The model under review builds one solid part; all positions refer to its coordinate system, in mm. Face numbers are marked on the shaded views. A direction names the side the tool comes from. Round coordinates to 2 decimals unless told otherwise and drop trailing zeros. Loops run counter-clockwise (first coordinate to the right, second up) from the corner with the lowest first, then second, coordinate; pieces in that order, holes last. Notation, with made-up numbers: M 30,84 L 36,84 A12 ccw 36,97 Z; hole C 69.5,51 d7. An arc over 180 degrees is marked long. Answer as a JSON object with one key per item and string values. Group by question number.
Item 1: Consider section A-A (y = 602.5). Give the boundary of the cut face in (x, z) (3 decimals), and give its area (3 significant figures).
Item 2: Consider section B-B (x = 34). Give the boundary of the cut face in (y, z), and give its area (3 significant figures).
Item 3: Insertion check: P1, Ø12, axis at y = -65, z = 20.5, coming from the +X side; P2, Ø1, axis at x = 56, y = 203, coming from the +Z side. Each pin has a flat end and moves straight along its axis. Give the tip position at first contact, or say it passes through.
Item 4: Tool access review of the marked faces 1 and 2: name each direction out of +Z, -Z, +X, -X, +Y, -Y from which nothing blocks a thin tool from reaching the whole face with its end or side.
Item 5: To check wall thickness, follow line 1 (Z direction, x = 1, y = -304); line 2 (X direction, y = 101.6, z = 4); line 3 (X direction, y = -406.4, z = 4.25). State the ranges of each line that lie inside material, in increasing order.
```python
from build123d import *

# Parameters (mm, degrees)
F1_DEPTH = 1066.8
F2_R     = 8.73125
F3_DEPTH = 76.201
F4_R     = 6.35
F5_DEPTH = 101.601


with BuildPart() as f1:
    # F0 (on Front) → F1 (new body, symmetric)
    with BuildSketch(Plane.XZ):
        with BuildLine():
            Line((3.175, 76.2), (0, 76.2))
            Line((0, 76.2), (0, 0))
            Line((0, 0), (101.6, 0))
            Line((101.6, 0), (101.6, 3.175))
            ThreePointArc((101.6, 3.175), (100.6700640303, 5.4200640303), (98.425, 6.35))
            Line((98.425, 6.35), (9.525, 6.35))
            ThreePointArc((9.525, 6.35), (7.2799359697, 7.2799359697), (6.35, 9.525))
            Line((6.35, 9.525), (6.35, 73.025))
            ThreePointArc((6.35, 73.025), (5.4200640303, 75.2700640303), (3.175, 76.2))
        make_face()
    extrude(amount=F1_DEPTH, both=True)

    # F2 (on face) → F3 (cut, through all)
    with BuildSketch(Plane(origin=(0, 0, 0), x_dir=(1, 0, 0), z_dir=(0, 0, -1))):
        with Locations((63.5, -203.2)):
            Circle(F2_R)
        with Locations((63.5, -406.4)):
            Circle(F2_R)
        with Locations((63.5, -101.6)):
            Circle(F2_R)
        with Locations((63.5, 101.6)):
            Circle(F2_R)
        with Locations((63.5, 203.2)):
            Circle(F2_R)
        with Locations((63.5, 406.4)):
            Circle(F2_R)
    extrude(amount=-F3_DEPTH, mode=Mode.SUBTRACT)

    # F4 (on face) → F5 (cut, through all)
    with BuildSketch(Plane(origin=(0, 0, 0), x_dir=(0, -1, 0), z_dir=(-1, 0, 0))):
        with Locations((-304.8, 41.275)):
            Circle(F4_R)
        with Locations((304.8, 41.275)):
            Circle(F4_R)
        with Locations((-914.4, 38.1)):
            Circle(F4_R)
        with Locations((914.4, 41.275)):
            Circle(F4_R)
    extrude(amount=-F5_DEPTH, mode=Mode.SUBTRACT)


solid = f1.part
```
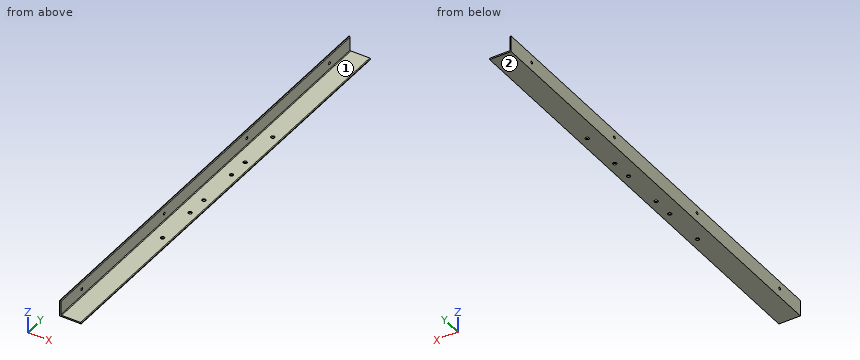
Geometry results:
{
 "1": {"outline": "M 0,0 L 101.6,0 L 101.6,3.175 A3.175 ccw 98.425,6.35 L 9.525,6.35 A3.175 cw 6.35,9.525 L 6.35,73.025 A3.175 ccw 3.175,76.2 L 0,76.2 Z", "area": "1,090 mm^2"},
 "2": {"outline": "M -1066.8,0 L 1066.8,0 L 1066.8,6.35 L -1066.8,6.35 Z", "area": "13,500 mm^2"},
 "3": {"P1": "stops at x = 6.35", "P2": "passes through"},
 "4": {"face 1": "+Z, +X, +Y, -Y", "face 2": "-Z, +X, -X, +Y, -Y"},
 "5": {"line 1": "z = 0 to 34.98, 47.57 to 76.2", "line 2": "x = 0 to 54.77, 72.23 to 101.49", "line 3": "x = 0 to 54.77, 72.23 to 101.41"}
}
